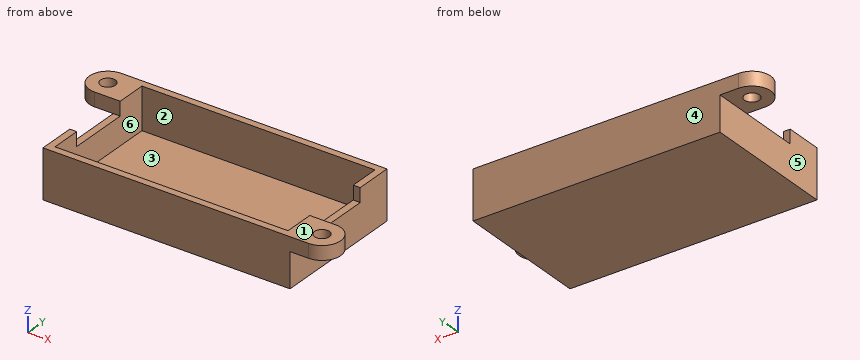
```python
from build123d import *

# Parameters (mm, degrees)
SKETCH_1_W          = 53
SKETCH_1_H          = 29
EXTRUDE_1_DEPTH     = 10.5
SHELL_1_T           = -1.5
SKETCH_3_R          = 1.6
EXTRUDE_2_DEPTH     = 3
SKETCH_4_W          = 3
SKETCH_4_H          = 13
CUT_EXTRUDE_1_DEPTH = 53


with BuildPart() as part:
    # 草图1 → 凸台-拉伸1 (new body)
    with BuildSketch(Plane.XY):
        Rectangle(SKETCH_1_W, SKETCH_1_H)
    extrude(amount=EXTRUDE_1_DEPTH)

    # 抽壳1
    shell_1_openings = [part.faces().sort_by_distance(p)[0] for p in [
        (0, 0, 10.5),
    ]]
    offset(amount=SHELL_1_T, openings=shell_1_openings, kind=Kind.INTERSECTION)

    # 草图3 → 凸台-拉伸2 (add)
    # profile 1 of 2: a face of its own
    with BuildSketch(Plane.XY.offset(10.5)):
        with BuildLine():
            Line((-26.5, 6.5), (-30.5, 6.5))
            ThreePointArc((-30.5, 6.5), (-34.5, 10.5), (-30.5, 14.5))
            Line((-30.5, 14.5), (-26.5, 14.5))
            Line((-26.5, 14.5), (-26.5, 6.5))
        make_face()
        with Locations((-30.5, 10.5)):
            Circle(SKETCH_3_R, mode=Mode.SUBTRACT)
    # profile 2 of 2: a face of its own
    with BuildSketch(Plane.XY.offset(10.5)):
        with BuildLine():
            Line((26.5, -6.5), (30.5, -6.5))
            ThreePointArc((30.5, -6.5), (34.5, -10.5), (30.5, -14.5))
            Line((30.5, -14.5), (26.5, -14.5))
            Line((26.5, -14.5), (26.5, -6.5))
        make_face()
        with Locations((30.5, -10.5)):
            Circle(SKETCH_3_R, mode=Mode.SUBTRACT)
    extrude(amount=-EXTRUDE_2_DEPTH)

    # 草图4 → 切除-拉伸1 (cut)
    with BuildSketch(Plane.ZY.offset(26.5)):
        with Locations((9, 0)):
            Rectangle(SKETCH_4_W, SKETCH_4_H)
    extrude(amount=-CUT_EXTRUDE_1_DEPTH, mode=Mode.SUBTRACT)


solid = part.part
```
Build history of the part. All positions in model axes, mm. Face numbers are marked on the shaded views. A direction names the side the tool comes from. Coordinates: 2 decimals unless noted, no trailing zeros. Order: outer loops, then holes, each group sorted by start corner. A loop starts at its lowest first (then second) coordinate and runs counter-clockwise, first axis right, second up. Notation, with made-up numbers: (2, 2.25) -> (42, 2.25) arc R19 cw to (42, 24.25) -> close; hole circle Ø4 at (-30, 22.5). An arc over 180 degrees is marked (long way). Answer in a Markdown table with one row per item. Add a question column.
Q1. Band-saw the part on A-A, the plane y = 10.5. List the corners of the cut face in (x, z), then the cut area to 3 significant figures.
Q2. Band-saw the part on B-B, the plane z = 2.25. List the corners of the cut face in (x, y).
Q3. Drop flat-ended pins along their axis: pin 1 (2.5 mm diameter, centred on x = -30.5, y = 10.5, fed in from +Z); pin 2 (2 mm diameter, centred on y = -8, z = 1.5, fed in from -X); pin 3 (1.2 mm diameter, centred on x = 26, y = -1.5, fed in from +Z); pin 4 (3.5 mm diameter, centred on x = 29, z = 8.5, fed in from +Y). Give the stop position or say it passes through.
Q4. Wall check: line 1 along Y through (x, z) = (-14.5, 2.5); line 2 along X through (y, z) = (5.5, 2.5); line 3 along Y through (x, z) = (-30.5, 8.15). Give the ranges that are in metal, low to high. Write a range as [from, to].
Q5. Mould opens along X. For the marked faces 3, 4, 5 and 6 say: +X half, -X half, draft (parallel to the pull), parting line (faces both ways), or undercut.
Q6. Which spindle directions (+Z, -Z, +X, -X, +Y, -Y) get a long thin tool onto all of the face, cutting with end or side? Do the marked faces 1 and 2. Say none if no direction does.
Q7. Band-saw the part on C-C, the plane y = 4.5. List the corners of the cut face in (x, z).
Q8. Band-saw the part on D-D, the plane x = 24. List the corners of the cut face in (y, z), then the cut area to 3 significant figures.
Answers follow:
| question | item | result |
|---|---|---|
| 1 | outline | (-34.5, 7.5) -> (-32.1, 7.5) -> (-32.1, 10.5) -> (-34.5, 10.5) -> close; (-28.9, 7.5) -> (-26.5, 7.5) -> (-26.5, 0) -> (26.5, 0) -> (26.5, 10.5) -> (25, 10.5) -> (25, 1.5) -> (-25, 1.5) -> (-25, 10.5) -> (-28.9, 10.5) -> close |
| 1 | area | 121 mm^2 |
| 2 | outline | (-26.5, -14.5) -> (26.5, -14.5) -> (26.5, 14.5) -> (-26.5, 14.5) -> close; hole (-25, -13) -> (25, -13) -> (25, 13) -> (-25, 13) -> close |
| 3 | pin 1 | through |
| 3 | pin 2 | x = -26.5 |
| 3 | pin 3 | z = 7.5 |
| 3 | pin 4 | y = -6.5 |
| 4 | line 1 | [-14.5, -13], [13, 14.5] |
| 4 | line 2 | [-26.5, -25], [25, 26.5] |
| 4 | line 3 | [6.5, 8.9], [12.1, 14.5] |
| 5 | face 3 | undercut |
| 5 | face 4 | draft |
| 5 | face 5 | -X half |
| 5 | face 6 | undercut |
| 6 | face 1 | +Z, +X, -X, +Y, -Y |
| 6 | face 2 | +Z |
| 7 | outline | (-26.5, 0) -> (26.5, 0) -> (26.5, 7.5) -> (25, 7.5) -> (25, 1.5) -> (-25, 1.5) -> (-25, 7.5) -> (-26.5, 7.5) -> close |
| 8 | outline | (-14.5, 0) -> (14.5, 0) -> (14.5, 10.5) -> (13, 10.5) -> (13, 1.5) -> (-13, 1.5) -> (-13, 10.5) -> (-14.5, 10.5) -> close |
| 8 | area | 70.5 mm^2 |
